The listing builds one solid part. Answer for the finished solid, in the listing's coordinates (mm). A direction names the side the tool comes from. Round coordinates to 2 decimals unless told otherwise and drop trailing zeros. Order: outer loops, then holes, each group sorted by start corner. A loop starts at its lowest first (then second) coordinate and runs counter-clockwise, first axis right, second up. Notation, with made-up numbers: M -20.5,11 L 32.5,11 A24 ccw 32.5,37 Z; hole C 9.25,-34.75 d4. An arc over 180 degrees is marked long. Put each result on its own line as item: value. Start each with the question number.
1. The mould has two halves that part along X. Classify faces 3 (the face through (-5, -3.5, 10)), 4 (the face through (16.15, 10, 0)), 5 (the face through (10.488, -1.726, -10.108)): +X half, -X half, draft (parallel to the pull), parting line (faces both ways), or undercut.
2. The part is cut by section D-D (z = 4.75). Give the vertices of the cut face in (x, y).
3. Each of these flat-tipped pins is pushed along its axis until it touches: pin 1 Ø1 at (y, z) = (-1, 0) entering from +X; pin 2 Ø2 at (x, z) = (4, -0.5) entering from -Y. Where does it stop, or does it pass through?
4. Which of the six approach directions +Z, -Z, +X, -X, +Y, -Y give full straight-line access (tool end or side, diameter ignored) to faces 1 (the face through (-9.512, -1.726, -10.108)), 2 (the face through (-10, -3.5, -10))?
5. Consider line 1 (Y direction, x = 13.5, z = 4.25). Determine where the line is inside the solid, lowest interval first.
6. The part is cut by section B-B (x = -10). Give the vertices of the cut face in (y, z).
7. The part is cut by section A-A (z = -10). Give the vertices of the cut face in (x, y), then the cut area to 3 significant figures.
8. The part is cut by section C-C (x = 1). Give the vertices of the cut face in (y, z).
from build123d import *

# Parameters (mm, degrees)
SKETCH1_W            = 32.3
SKETCH1_H            = 27.3
BASE_EXTRUSION_DEPTH = 20
SKETCH2_R            = 0.5
PINS_DEPTH           = 3.5


with BuildPart() as part:
    # Sketch1 → Base Extrusion (new body)
    with BuildSketch(Plane(origin=(0, 0, 0), x_dir=(1, 0, 0), z_dir=(0, 1, 0))):
        Rectangle(SKETCH1_W, SKETCH1_H)
    extrude(amount=BASE_EXTRUSION_DEPTH)

    # Sketch2 → Pins (add)
    with BuildSketch(Plane.XZ):
        with Locations(Location((-5, 10, 0), (0, 0, 90))):
            Circle(SKETCH2_R)
        with Locations(Location((5, 10, 0), (0, 0, 90))):
            Circle(SKETCH2_R)
        with Locations(Location((-10, -10, 0), (0, 0, 90))):
            Circle(SKETCH2_R)
        with Locations(Location((10, -10, 0), (0, 0, 90))):
            Circle(SKETCH2_R)
    extrude(amount=PINS_DEPTH)


solid = part.part
Resolved:
1. face 3: draft
1. face 4: +X half
1. face 5: undercut
2. outline: M -16.15,0 L 16.15,0 L 16.15,20 L -16.15,20 Z
3. pin 1: through
3. pin 2: y = 0
4. face 1: -Y
4. face 2: +Z, -Z, +X, -X, -Y
5. line 1: 0 to 20
6. outline: M -3.5,-10.5 L 0,-10.5 L 0,-13.65 L 20,-13.65 L 20,13.65 L 0,13.65 L 0,-9.5 L -3.5,-9.5 Z
7. outline: M -16.15,0 L -10.5,0 L -10.5,-3.5 L -9.5,-3.5 L -9.5,0 L 9.5,0 L 9.5,-3.5 L 10.5,-3.5 L 10.5,0 L 16.15,0 L 16.15,20 L -16.15,20 Z
7. area: 653 mm2
8. outline: M 0,-13.65 L 20,-13.65 L 20,13.65 L 0,13.65 Z
